For this review, take the finished solid that the model builds, in its own axes (mm). A direction names the side the tool comes from. Round coordinates to 2 decimals unless told otherwise and drop trailing zeros. Write each loop counter-clockwise with the first axis right and the second up, starting at its lowest first coordinate (ties: lowest second). Pieces come first, ordered by that corner, then holes. Notation, with made-up numbers: M 48.5,-4.75 L 77.5,-4.75 A8 ccw 77.5,-0.75 Z; hole C 41.25,14 d1. An arc over 180 degrees is marked long. Use one line per item in the form item = value. Start each with the question number.
Item 1: For line 1 (X direction, y = -0.5, z = -3) (3 decimals); line 2 (X direction, y = -3.75, z = 2.25) (3 decimals); line 3 (Y direction, x = -9, z = -3), list the stretches that pass through material, from the lowest coordinate up. Write a range as [from, to].
Item 2: Add section D-D (x = 0.5). State the section outline as (y, z) points (3 decimals).
Item 3: For P1, Ø0.6, axis at x = 6.5, y = -4.5, coming from the +Z side (3 decimals); P2, Ø2, axis at x = 5, y = -4.5, coming from the -Z side (3 decimals); P3, Ø8, axis at x = 3, z = 10.5, coming from the +Y side; P4, Ø6, axis at x = 1, y = 2.5, coming from the +Z side (3 decimals), all flat-tipped, find the tip position at first contact; note any pin that passes through.
Item 4: Add section B-B (y = -1.5). State the section outline as (x, z) points (3 decimals), and give its area (3 significant figures).
Item 5: Add section C-C (z = -2.5). State the section outline as (x, y) points (3 decimals), and give its area (3 significant figures).
Item 6: Add section A-A (x = 6.5). State the section outline as (y, z) points (3 decimals), and give its area (3 significant figures).
Item 7: Draft analysis for pull direction X (two halves, no side actions). For faces 1 (the flat face through (0, -2, -1.955)), 2 (the flat face through (0, 0, -5)), 3 (the flat face through (-5, -4.915, 4)), 4 (the flat face through (7.855, -4, 4)), state which applies: released by +X, released by -X, zero draft, split by the parting line, or undercut.
Item 8: For faces 5 (the flat face through (2.005, -4, 4)), 6 (the flat face through (8.95, 4, -7)), 7 (the flat face through (-7.855, -4, 4)), list the 3-axis set-ups (+Z, -Z, +X, -X, +Y, -Y) from which the entire face can be reached by the end or side of a thin tool; tool diameter is ignored.
from build123d import *

# Parameters (mm, degrees)
SKETCH_1_W          = 22.81
SKETCH_1_H          = 17.75
EXTRUDE_1_DEPTH     = 1.06
SKETCH_2_W          = 1.44
SKETCH_2_H          = 3.065036756
EXTRUDE_2_DEPTH     = 6.92
EXTRUDE_3_DEPTH     = 3.065036756
SKETCH_4_R          = 2.925
EXTRUDE_4_DEPTH     = 5.85
SKETCH_5_W          = 22.81
SKETCH_5_H          = 4.28
EXTRUDE_5_DEPTH     = 5.53
SKETCH_6_R          = 1.75
CUT_EXTRUDE_1_DEPTH = 5.53
SKETCH_7_W          = 14
SKETCH_7_H          = 6
EXTRUDE_6_DEPTH     = 4.125036756
CUT_EXTRUDE_START   = -4
SKETCH_8_R          = 2.925
CUT_EXTRUDE_2_DEPTH = 4
EXTRUDE_START       = -1.85
EXTRUDE_7_DEPTH     = 1.85
SKETCH_10_W         = 2.455
SKETCH_10_H         = 4.28
CUT_EXTRUDE_3_DEPTH = 5.53


with BuildPart() as part:
    # 草图1 → 凸台-拉伸1 (new body)
    with BuildSketch(Plane(origin=(0, 0, 0), x_dir=(1, 0, 0), z_dir=(0, 1, 0))):
        Rectangle(SKETCH_1_W, SKETCH_1_H)
    extrude(amount=EXTRUDE_1_DEPTH)

    # 草图2 → 凸台-拉伸2 (add)
    with BuildSketch(Plane(origin=(0, 0, -8.875), x_dir=(-1, 0, 0), z_dir=(0, 0, -1))):
        with Locations((-10.685, -1.532518378)):
            Rectangle(SKETCH_2_W, SKETCH_2_H)
        with Locations((10.685, -1.532518378)):
            Rectangle(SKETCH_2_W, SKETCH_2_H)
    extrude(amount=-EXTRUDE_2_DEPTH)

    # 草图3 → 凸台-拉伸3 (add)
    with BuildSketch(Plane.XZ):
        Polygon((-11.405, 8.875), (-11.405, -1.955), (-9.965, -1.955), (9.965, -1.955), (11.405, -1.955), (11.405, 8.875), align=None)
    extrude(amount=EXTRUDE_3_DEPTH)

    # 草图4 → 凸台-拉伸4 (add)
    with BuildSketch(Plane.XZ.offset(3.065036756)):
        with Locations(Location((-4.93, 3.75, 0), (0, 0, 270))):
            Circle(SKETCH_4_R)
        with Locations(Location((4.93, 3.75, 0), (0, 0, 270))):
            Circle(SKETCH_4_R)
    extrude(amount=EXTRUDE_4_DEPTH)

    # 草图5 → 凸台-拉伸5 (add)
    with BuildSketch(Plane(origin=(0, 1.06, 0), x_dir=(1, 0, 0), z_dir=(0, 1, 0))):
        with Locations((0, 6.735)):
            Rectangle(SKETCH_5_W, SKETCH_5_H)
    extrude(amount=EXTRUDE_5_DEPTH)

    # 草图6 → 切除-拉伸1 (cut)
    with BuildSketch(Plane.XY.offset(-4.595)):
        with Locations((5.535, 3.825)):
            Circle(SKETCH_6_R)
        with Locations((-5.535, 3.825)):
            Circle(SKETCH_6_R)
    extrude(amount=-CUT_EXTRUDE_1_DEPTH, mode=Mode.SUBTRACT)

    # 草图7 → 凸台-拉伸6 (add)
    with BuildSketch(Plane(origin=(0, 1.06, 0), x_dir=(1, 0, 0), z_dir=(0, 1, 0))):
        with Locations((0, -11.875)):
            Rectangle(SKETCH_7_W, SKETCH_7_H)
    extrude(amount=-EXTRUDE_6_DEPTH)

    # 草图8 → 切除-拉伸2 (cut)
    with BuildSketch(Plane.XZ.offset(8.915036756).offset(CUT_EXTRUDE_START)):
        with Locations(Location((-4.93, 3.75, 0), (0, 0, 270))):
            Circle(SKETCH_8_R)
        with Locations(Location((4.93, 3.75, 0), (0, 0, 270))):
            Circle(SKETCH_8_R)
    extrude(amount=CUT_EXTRUDE_2_DEPTH, mode=Mode.SUBTRACT)

    # 草图9 → 凸台-拉伸7 (add)
    with BuildSketch(Plane.XZ.offset(4.915036756).offset(EXTRUDE_START)):
        with BuildLine():
            ThreePointArc((-7.855, 3.75), (-6.998287335, 5.818287335), (-4.93, 6.675))
            Line((-4.93, 6.675), (-7.855, 6.675))
            Line((-7.855, 6.675), (-7.855, 3.75))
        make_face()
        with BuildLine():
            Line((-7.855, 0.825), (-4.93, 0.825))
            ThreePointArc((-4.93, 0.825), (-6.998287335, 1.681712665), (-7.855, 3.75))
            Line((-7.855, 3.75), (-7.855, 0.825))
        make_face()
        with BuildLine():
            Line((-2.005, 0.825), (-2.005, 3.75))
            ThreePointArc((-2.005, 3.75), (-2.861712665, 1.681712665), (-4.93, 0.825))
            Line((-4.93, 0.825), (-2.005, 0.825))
        make_face()
        with BuildLine():
            ThreePointArc((-4.93, 6.675), (-2.861712665, 5.818287335), (-2.005, 3.75))
            Line((-2.005, 3.75), (-2.005, 6.675))
            Line((-2.005, 6.675), (-4.93, 6.675))
        make_face()
        with BuildLine():
            ThreePointArc((2.005, 3.75), (2.861712665, 5.818287335), (4.93, 6.675))
            Line((4.93, 6.675), (2.005, 6.675))
            Line((2.005, 6.675), (2.005, 3.75))
        make_face()
        with BuildLine():
            ThreePointArc((4.93, 0.825), (2.861712665, 1.681712665), (2.005, 3.75))
            Line((2.005, 3.75), (2.005, 0.825))
            Line((2.005, 0.825), (4.93, 0.825))
        make_face()
        with BuildLine():
            Line((7.855, 0.825), (7.855, 3.75))
            ThreePointArc((7.855, 3.75), (6.998287335, 1.681712665), (4.93, 0.825))
            Line((4.93, 0.825), (7.855, 0.825))
        make_face()
        with BuildLine():
            Line((7.855, 6.675), (4.93, 6.675))
            ThreePointArc((4.93, 6.675), (6.998287335, 5.818287335), (7.855, 3.75))
            Line((7.855, 3.75), (7.855, 6.675))
        make_face()
    extrude(amount=EXTRUDE_7_DEPTH)

    # 草图10 → 切除-拉伸3 (cut)
    with BuildSketch(Plane(origin=(0, 6.59, 0), x_dir=(1, 0, 0), z_dir=(0, 1, 0))):
        with Locations((-10.1775, 6.735)):
            Rectangle(SKETCH_10_W, SKETCH_10_H)
        with Locations((10.1775, 6.735)):
            Rectangle(SKETCH_10_W, SKETCH_10_H)
    extrude(amount=-CUT_EXTRUDE_3_DEPTH, mode=Mode.SUBTRACT)


solid = part.part
Calculated:
q1.line_1 = [-11.405, -9.965], [9.965, 11.405]
q1.line_2 = [-7.855, -2.005], [2.005, 7.855]
q1.line_3 = [0, 1.06]
q2.outline = M -3.065,-1.955 L 0,-1.955 L 0,-8.875 L 6.59,-8.875 L 6.59,-4.595 L 1.06,-4.595 L 1.06,14.875 L -3.065,14.875 Z
q3.P1 = 6.675
q3.P2 = 0.825
q3.P3 = 1.06
q3.P4 = 14.875
q4.outline = M -11.405,-8.875 L -9.965,-8.875 L -9.965,-1.955 L 9.965,-1.955 L 9.965,-8.875 L 11.405,-8.875 L 11.405,8.875 L 7,8.875 L 7,14.875 L -7,14.875 L -7,8.875 L -11.405,8.875 Z
q4.area = 351 mm^2
q5.outline = M -11.405,-3.065 L -9.965,-3.065 L -9.965,0 L 9.965,0 L 9.965,-3.065 L 11.405,-3.065 L 11.405,1.06 L -11.405,1.06 Z
q5.area = 33.0 mm^2
q6.outline = M -4.915,0.825 L -3.065,0.825 L -3.065,-1.955 L 0,-1.955 L 0,-8.875 L 2.365,-8.875 L 2.365,-4.595 L 1.06,-4.595 L 1.06,14.875 L -3.065,14.875 L -3.065,6.675 L -4.915,6.675 Z; M 5.285,-8.875 L 6.59,-8.875 L 6.59,-4.595 L 5.285,-4.595 Z
q6.area = 98.8 mm^2
q7.face_1 = undercut
q7.face_2 = undercut
q7.face_3 = zero draft
q7.face_4 = released by +X
q8.face_5 = +Z, -Z, -Y
q8.face_6 = +Z, -Z, +X, +Y
q8.face_7 = +Z, -Z, -X, -Y
